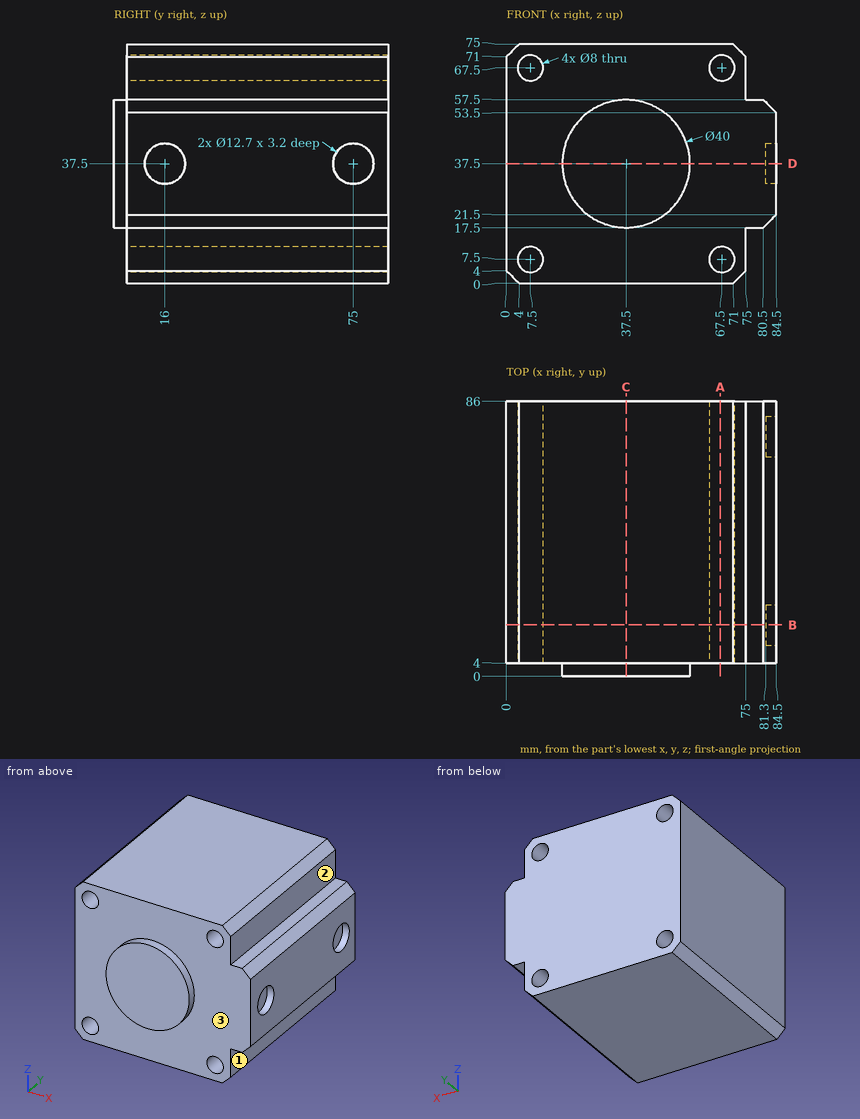
Geometry check sheet. Reference: drawing and pictorial views, mm from the part's lowest x, y, z. A direction names the side the tool comes from. Give positions to 0.01 mm unless a question says otherwise; leave off trailing zeros. Loops run counter-clockwise (first coordinate to the right, second up) from the corner with the lowest first, then second, coordinate; pieces in that order, holes last.
1. Thickness scan on line 1 (Y direction, x = 83.05, z = 37.5); line 2 (Z direction, x = 67.5, y = 36); line 3 (X direction, y = 64, z = 6). Record the ranges inside material, lowest first.
2. Go/stop test with flat-tipped pins: pin 1 Ø5 at (x, z) = (35, 8.5) entering from -Y; pin 2 Ø7 at (x, z) = (67.5, 67.5) entering from +Y; pin 3 Ø6 at (x, y) = (77, 56.5) entering from -Z; pin 4 Ø3 at (x, y) = (79, 37.5) entering from +Z. Record where each tip stops, or that it passes through.
3. Set-up check for the marked faces 1, 2 and 3: record each of +Z, -Z, +X, -X, +Y, -Y from which the full face is reachable in a straight line by a thin tool's end or side.
4. Section check C-C, the plane x = 37.5. Enter the section's corners in (y, z), then the cut area to 3 significant figures.
5. Section check B-B, the plane y = 16. Enter the section's corners in (x, z), then the cut area to 3 significant figures.
6. Section check D-D, the plane z = 37.5. Enter the section's corners in (x, y).
7. Section check A-A, the plane x = 67. Enter the section's corners in (y, z), then the cut area to 3 significant figures.
Geometry says:
1. line 1: y = 4 to 9.65, 22.35 to 68.65, 81.35 to 86
1. line 2: z = 0 to 3.5, 11.5 to 63.5, 71.5 to 75
1. line 3: x = 0 to 3.79, 11.21 to 63.79, 71.21 to 75
2. pin 1: stops at y = 4
2. pin 2: passes through
2. pin 3: stops at z = 3
2. pin 4: stops at z = 57.5
3. face 1: -Z, +X, +Y, -Y
3. face 2: +Z, +X, +Y, -Y
3. face 3: -Y
4. outline: (0, 17.5) - (4, 17.5) - (4, 0) - (86, 0) - (86, 75) - (4, 75) - (4, 57.5) - (0, 57.5) - close
4. area: 6,310 mm2
5. outline: (0, 4) - (4, 0) - (71, 0) - (75, 4) - (75, 17.5) - (80.5, 17.5) - (84.5, 21.5) - (84.5, 31.15) - (81.3, 31.15) - (81.3, 43.85) - (84.5, 43.85) - (84.5, 53.5) - (80.5, 57.5) - (75, 57.5) - (75, 71) - (71, 75) - (4, 75) - (0, 71) - close; hole circle Ø8 at (7.5, 7.5); hole circle Ø8 at (7.5, 67.5); hole circle Ø8 at (67.5, 7.5); hole circle Ø8 at (67.5, 67.5)
5. area: 5,720 mm2
6. outline: (0, 4) - (17.5, 4) - (17.5, 0) - (57.5, 0) - (57.5, 4) - (84.5, 4) - (84.5, 9.65) - (81.3, 9.65) - (81.3, 22.35) - (84.5, 22.35) - (84.5, 68.65) - (81.3, 68.65) - (81.3, 81.35) - (84.5, 81.35) - (84.5, 86) - (0, 86) - close
7. outline: (4, 0) - (86, 0) - (86, 3.53) - (4, 3.53) - close; (4, 11.47) - (86, 11.47) - (86, 63.53) - (4, 63.53) - close; (4, 71.47) - (86, 71.47) - (86, 75) - (4, 75) - close
7. area: 4,850 mm2
